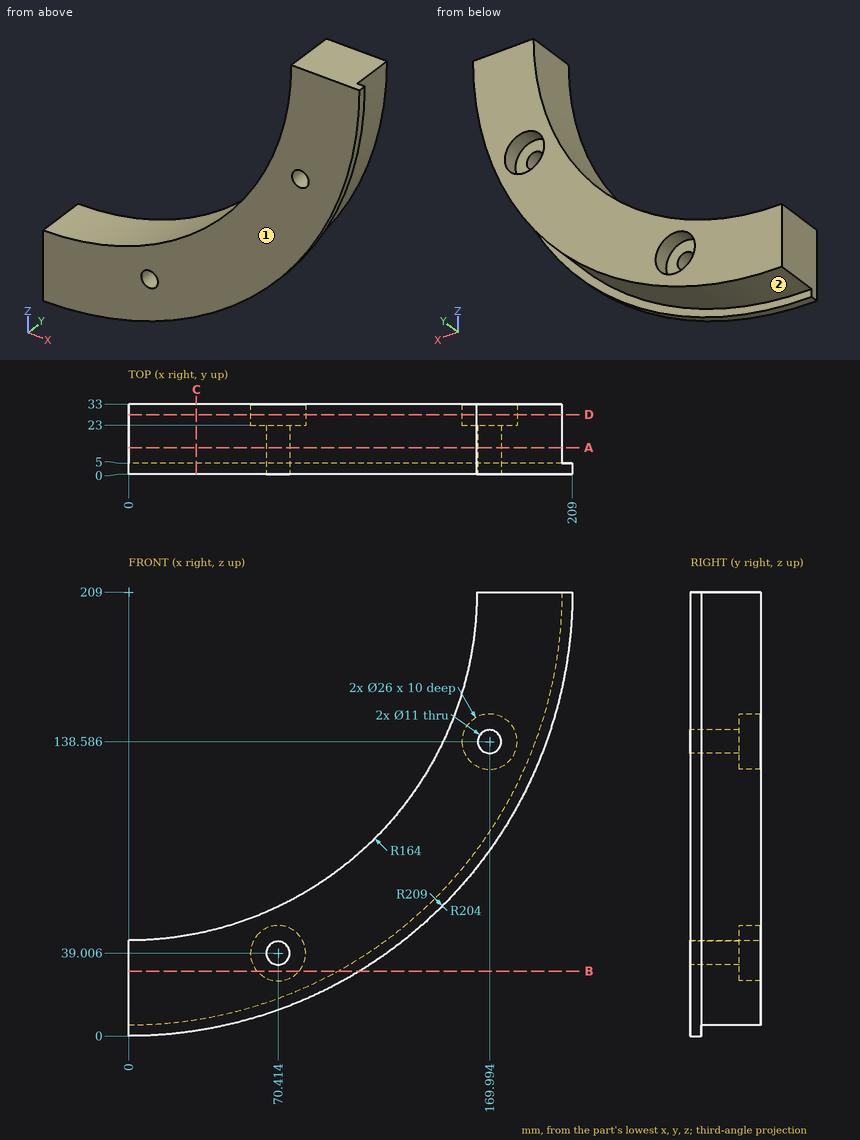
Study the drawing (mm; zero at the part's minimum x, y, z) and answer. A direction names the side the tool comes from. Give positions to 0.01 mm unless a question says otherwise; leave off trailing zeros. Write each loop counter-clockwise with the first axis right and the second up, starting at its lowest first coordinate (ties: lowest second). Pieces come first, ordered by that corner, then holes.
(1) Which of the six approach directions +Z, -Z, +X, -X, +Y, -Y give full straight-line access (tool end or side, diameter ignored) to the marked faces 1 and 2?
Final values:
face 1: +Z, -Z, +X, -X, -Y
face 2: -Z, +X, +Y
(2) The part is cut by section A-A on y = 12.5. Write down the section's boundary in (x, z) (1 decimal).
Final values:
outline: (0, 5) arc R204 ccw to (204, 209) - (164, 209) arc R164 cw to (0, 45) - close; hole circle Ø11 at (70.4, 39); hole circle Ø11 at (170, 138.6)
(3) The part is cut by section C-C on x = 32. Write down the section's boundary in (y, z) (1 decimal), plus the area to 3 significant figures.
Final values:
outline: (0, 2.5) - (5, 2.5) - (5, 7.5) - (33, 7.5) - (33, 48.2) - (0, 48.2) - close
area: 1,370 mm2
(4) Flat-ended cylindrical pins translate along their axes: pin 1 Ø2 at (x, y) = (58, 21.5) entering from -Z (1 decimal); pin 2 Ø1 at (y, z) = (26, 77) entering from -X; pin 3 Ø13 at (x, z) = (171, 136) entering from +Y. Find the tip coordinate at first contact, or state that the pin passes through.
Final values:
pin 1: stops at z = 13.1
pin 2: stops at x = 96.64
pin 3: stops at y = 23
(5) The part is cut by section B-B on z = 30.5. Write down the section's boundary in (x, y) (1 decimal).
Final values:
outline: (0, 0) - (108.7, 0) - (108.7, 5) - (98.8, 5) - (98.8, 33) - (80.2, 33) - (80.2, 23) - (60.6, 23) - (60.6, 33) - (0, 33) - close
(6) The part is cut by section D-D on y = 28. Write down the section's boundary in (x, z), plus the area to 3 significant figures.
Final values:
outline: (0, 5) arc R204 ccw to (204, 209) - (164, 209) arc R164 cw to (0, 45) - close; hole circle Ø26 at (70.41, 39.01); hole circle Ø26 at (169.99, 138.59)
area: 10,500 mm2
(7) Straight lines are drawn through the part: line 1 (Z direction, x = 60.5, y = 25.5) (1 decimal); line 2 (Z direction, x = 178, y = 28) (1 decimal); line 3 (Z direction, x = 8, y = 7) (1 decimal). For each, find the intervals that lie inside material, in ascending order.
Final values:
line 1: z = 14.2 to 30.6, 47.4 to 56.6
line 2: z = 109.3 to 128.3, 148.8 to 209
line 3: z = 5.2 to 45.2
